```python
from build123d import *

# Parameters (mm, degrees)
SKETCH1_W               = 488
SKETCH1_H               = 25
SKETCH1_R               = 7.5
BOSS_EXTRUDE1_DEPTH     = 25
CUT_EXTRUDE1_DEPTH      = 489.799805646
CUT_EXTRUDE1_DEPTH_BACK = 489.799805646
SKETCH2_W               = 12.5
SKETCH2_H               = 25


with BuildPart() as part:
    # Sketch1 → Boss-Extrude1 (new body)
    with BuildSketch(Plane.XY):
        Rectangle(SKETCH1_W, SKETCH1_H)
        with Locations((-224, 0)):
            Circle(SKETCH1_R, mode=Mode.SUBTRACT)
        with Locations((224, 0)):
            Circle(SKETCH1_R, mode=Mode.SUBTRACT)
    extrude(amount=BOSS_EXTRUDE1_DEPTH)

    # Sketch2 → Cut-Extrude1 (cut, two sides: drawn at the far end of the back side and taken through both)
    with BuildSketch(Plane(origin=(244, 0, 0), x_dir=(0, 0, -1), z_dir=(1, 0, 0)).offset(-CUT_EXTRUDE1_DEPTH_BACK)):
        with Locations((-6.25, 0)):
            Rectangle(SKETCH2_W, SKETCH2_H)
    extrude(amount=CUT_EXTRUDE1_DEPTH + CUT_EXTRUDE1_DEPTH_BACK, mode=Mode.SUBTRACT)


solid = part.part
```
Input: part model. Units: mm. Frame: model coordinates. Round coordinates to 2 decimals unless told otherwise and drop trailing zeros. Loops run counter-clockwise (first coordinate to the right, second up) from the corner with the lowest first, then second, coordinate; pieces in that order, holes last.
1) Section query C-C on z = 21.5. Return the cut outline in (x, y).
Ans:
outline: (-244, -12.5) - (244, -12.5) - (244, 12.5) - (-244, 12.5) - close; hole circle Ø15 at (-224, 0); hole circle Ø15 at (224, 0)
2) Section query A-A on y = 0. Return the cut outline in (x, z).
Ans:
outline: (-244, 12.5) - (-231.5, 12.5) - (-231.5, 25) - (-244, 25) - close; (-216.5, 12.5) - (216.5, 12.5) - (216.5, 25) - (-216.5, 25) - close; (231.5, 12.5) - (244, 12.5) - (244, 25) - (231.5, 25) - close
3) Section query B-B on x = 224. Return the cut outline in (y, z), plus the area to 3 significant figures.
Ans:
outline: (-12.5, 12.5) - (-7.5, 12.5) - (-7.5, 25) - (-12.5, 25) - close; (7.5, 12.5) - (12.5, 12.5) - (12.5, 25) - (7.5, 25) - close
area: 125 mm2
4) Material intervals for line 1 (X direction, y = 0.25, z = 21.75); line 2 (X direction, y = 1, z = 17); line 3 (Y direction, x = 224, z = 19.25), sorted ascending.
Ans:
line 1: x = -244 to -231.5, -216.5 to 216.5, 231.5 to 244
line 2: x = -244 to -231.43, -216.57 to 216.57, 231.43 to 244
line 3: y = -12.5 to -7.5, 7.5 to 12.5
5) Pin query (flat end, axial travel): pin 1 (13.5 mm diameter, centred on x = -224, y = 0, fed in from +Z). Return the tip coordinate at first contact, or that it passes through.
Ans:
pin 1: passes through
6) Pull-direction query (Y, two-part tool) for faces 1 (the flat face through (244, 0, 19)), 2 (the flat face through (-3, 12.5, 19)), 3 (the cylindrical face through (-231.493, 0.33, 18.662)), 4 (the flat face through (-3, -12.5, 19)); classes: released by +Y, released by -Y, zero draft, split by the parting line, or undercut.
Ans:
face 1: zero draft
face 2: released by +Y
face 3: undercut
face 4: released by -Y
